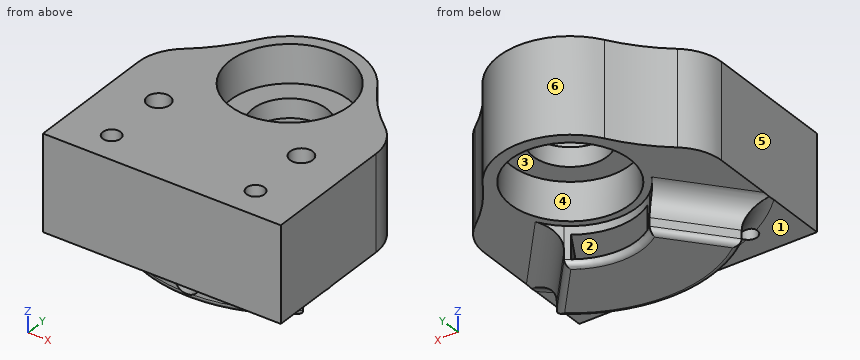
from build123d import *

# Parameters (mm, degrees)
EXTRUDE_1_DEPTH          = 4
EXTRUDE_1_DEPTH_BACK     = 4
SKETCH_2_R               = 0.95
SKETCH_2_R_2             = 0.75
SKETCH_3_R               = 5
CUT_EXTRUDE_1_DEPTH      = 3.2
SKETCH_6_R               = 3.1
CUT_EXTRUDE_2_DEPTH      = 24.749526311
EXTRUDE_3_DEPTH          = 3.2
CUT_EXTRUDE_3_DEPTH      = 1.2
CUT_EXTRUDE_3_DEPTH_BACK = 0.8
SKETCH_10_R              = 0.95
EXTRUDE_4_DEPTH          = 2
FILLET_4_R               = 2
FILLET_START             = -7
FILLET_5_2_DEPTH         = 9
FILLET_START_2           = -2
FILLET_5_3_DEPTH         = 9
SKETCH_11_R              = 1.1
CUT_EXTRUDE_4_DEPTH      = 5


with BuildPart() as part:
    # 草图2 → 凸台-拉伸1 (new, two sides: drawn at the far end of the back side and taken through both)
    with BuildSketch(Plane.XY.offset(-EXTRUDE_1_DEPTH_BACK)):
        with BuildLine():
            Line((-10, 11.178983643), (-10, 0))
            Line((-10, 0), (10, 0))
            Line((10, 0), (10, 11.178983643))
            ThreePointArc((10, 11.178983643), (9.606342006, 12.909387452), (8.502851331, 14.299197613))
            ThreePointArc((8.502851331, 14.299197613), (6.641519688, 16.075059286), (5.11101252, 18.142857143))
            ThreePointArc((5.11101252, 18.142857143), (0, 21), (-5.11101252, 18.142857143))
            ThreePointArc((-5.11101252, 18.142857143), (-6.641519688, 16.075059286), (-8.502851331, 14.299197613))
            ThreePointArc((-8.502851331, 14.299197613), (-9.606342006, 12.909387452), (-10, 11.178983643))
        make_face()
        with Locations((-6, 8)):
            Circle(SKETCH_2_R, mode=Mode.SUBTRACT)
        with Locations((-6.05, 2.55)):
            Circle(SKETCH_2_R_2, mode=Mode.SUBTRACT)
        with Locations(Location((6.05, 2.55, 0), (0, 0, 180))):
            Circle(SKETCH_2_R_2, mode=Mode.SUBTRACT)
        with Locations(Location((6, 8, 0), (0, 0, 180))):
            Circle(SKETCH_2_R, mode=Mode.SUBTRACT)
    extrude(amount=EXTRUDE_1_DEPTH + EXTRUDE_1_DEPTH_BACK)

    # 草图3 → 切除-拉伸1 (cut)
    with BuildSketch(Plane.XY.offset(4)):
        with Locations((0, 15)):
            Circle(SKETCH_3_R)
    cut_extrude_1 = extrude(amount=-CUT_EXTRUDE_1_DEPTH, mode=Mode.SUBTRACT)

    # 镜向1: 切除-拉伸1 across plane
    add(cut_extrude_1.mirror(Plane.XY), mode=Mode.SUBTRACT)

    # 草图6 → 切除-拉伸2 (cut, through all)
    with BuildSketch(Plane.XY.offset(0.8)):
        with Locations((0, 15)):
            Circle(SKETCH_6_R)
    extrude(amount=-CUT_EXTRUDE_2_DEPTH, mode=Mode.SUBTRACT)

    # 草图8 → 凸台-拉伸3 (add)
    with BuildSketch(Plane(origin=(0, 0, -4), x_dir=(-1, 0, 0), z_dir=(0, 0, -1))):
        with BuildLine():
            Line((-3.599610614, 10.710151119), (-7.777730077, 5.730862238))
            ThreePointArc((-7.777730077, 5.730862238), (0, 2.9), (7.777730077, 5.730862238))
            Line((7.777730077, 5.730862238), (3.599610614, 10.710151119))
            ThreePointArc((3.599610614, 10.710151119), (0, 9.4), (-3.599610614, 10.710151119))
        make_face()
    extrude(amount=EXTRUDE_3_DEPTH)

    # 草图9 → 切除-拉伸3 (cut, two sides: drawn at the far end of the back side and taken through both)
    with BuildSketch(Plane(origin=(0, 0, -5.5), x_dir=(-1, 0, 0), z_dir=(0, 0, -1)).offset(-CUT_EXTRUDE_3_DEPTH_BACK)):
        with BuildLine():
            Line((-3.221829655, 10.419627344), (-5.977379212, 5.646875508))
            ThreePointArc((-5.977379212, 5.646875508), (0, 3.9), (5.977379212, 5.646875508))
            Line((5.977379212, 5.646875508), (3.221829655, 10.419627344))
            ThreePointArc((3.221829655, 10.419627344), (0, 9.4), (-3.221829655, 10.419627344))
        make_face()
    extrude(amount=CUT_EXTRUDE_3_DEPTH + CUT_EXTRUDE_3_DEPTH_BACK, mode=Mode.SUBTRACT)

    # 草图10 → 凸台-拉伸4 (add)
    with BuildSketch(Plane(origin=(0, 0, -4), x_dir=(-1, 0, 0), z_dir=(0, 0, -1))):
        with Locations((-6, 8)):
            Circle(SKETCH_10_R)
        with Locations(Location((6, 8, 0), (0, 0, 180))):
            Circle(SKETCH_10_R)
    extrude(amount=-EXTRUDE_4_DEPTH)

    # 圆角4
    # the kernel refuses this fillet: 2 mm, written as the material it adds along each edge
    with BuildSketch(Plane(origin=(10.991668126, 1.900640023, -4), x_dir=(0.7660444431189769, 0.6427876096865407, 0), z_dir=(-0.6427876096865407, 0.7660444431189769, 0))) as fillet_4_piece_1_section:
        with BuildLine():
            CenterArc((FILLET_4_R, FILLET_4_R), FILLET_4_R, 180, 90)
            Line((0, FILLET_4_R), (0, 0))
            Line((0, 0), (FILLET_4_R, 0))
        make_face()
    fillet_4_piece_1 = extrude(amount=16.5, mode=Mode.PRIVATE)
    fillet_4_piece_1 = fillet_4_piece_1 - Plane(origin=(0, 15, -4), x_dir=(-0.6427876096865404, -0.7660444431189772, 0), z_dir=(0, 0, 1)) * Cylinder(5.6, 42, mode=Mode.PRIVATE)
    fillet_4_piece_1 = fillet_4_piece_1 & Plane(origin=(0, 15, -4), x_dir=(0.6427876096865403, -0.7660444431189773, 0), z_dir=(0, 0, 1)) * Cylinder(12.1, 42, mode=Mode.PRIVATE)
    add(fillet_4_piece_1)
    with BuildSketch(Plane(origin=(-0.385672566, 14.540373334, -4), x_dir=(-0.766044443118977, 0.6427876096865406, 0), z_dir=(-0.6427876096865406, -0.7660444431189771, 0))) as fillet_4_piece_2_section:
        with BuildLine():
            CenterArc((FILLET_4_R, FILLET_4_R), FILLET_4_R, 180, 90)
            Line((0, FILLET_4_R), (0, 0))
            Line((0, 0), (FILLET_4_R, 0))
        make_face()
    fillet_4_piece_2 = extrude(amount=16.5, mode=Mode.PRIVATE)
    fillet_4_piece_2 = fillet_4_piece_2 - Plane(origin=(0, 15, -4), x_dir=(-0.6427876096865404, -0.7660444431189772, 0), z_dir=(0, 0, 1)) * Cylinder(5.6, 42, mode=Mode.PRIVATE)
    fillet_4_piece_2 = fillet_4_piece_2 & Plane(origin=(0, 15, -4), x_dir=(0.6427876096865403, -0.7660444431189773, 0), z_dir=(0, 0, 1)) * Cylinder(12.1, 42, mode=Mode.PRIVATE)
    add(fillet_4_piece_2)
    with BuildSketch(Plane(origin=(0, 15, -4), x_dir=(0.6427876096865403, -0.7660444431189772, 0), z_dir=(0.7660444431189772, 0.6427876096865403, 0))) as fillet_4_piece_3_section:
        with BuildLine():
            CenterArc((12.1 + FILLET_4_R, FILLET_4_R), FILLET_4_R, 180, 90)
            Line((12.1, FILLET_4_R), (12.1, 0))
            Line((12.1, 0), (12.1 + FILLET_4_R, 0))
        make_face()
    fillet_4_piece_3 = revolve(axis=Axis((0, 15, -4), (0, 0, -1)), revolution_arc=80, mode=Mode.PRIVATE)
    fillet_4_piece_3 = fillet_4_piece_3 - Plane(origin=(-6.05, 2.55, -4), x_dir=(1, 0, 0), z_dir=(0, 0, -1)) * Cylinder(0.75, 57, mode=Mode.PRIVATE)
    fillet_4_piece_3 = fillet_4_piece_3 - Plane(origin=(6.05, 2.55, -4), x_dir=(-1, 0, 0), z_dir=(0, 0, -1)) * Cylinder(0.75, 57, mode=Mode.PRIVATE)
    add(fillet_4_piece_3)
    with BuildSketch(Plane(origin=(10.991668126, 1.900640023, -4), x_dir=(0.7660444431189769, 0.6427876096865407, 0), z_dir=(-0.6427876096865407, 0.7660444431189769, 0))) as fillet_4_piece_4a_section:
        with BuildLine():
            CenterArc((FILLET_4_R, FILLET_4_R), FILLET_4_R, 180, 90)
            Line((0, FILLET_4_R), (0, 0))
            Line((0, 0), (FILLET_4_R, 0))
        make_face()
    fillet_4_piece_4a = extrude(amount=16.5, mode=Mode.PRIVATE)
    fillet_4_piece_4a = split(fillet_4_piece_4a, bisect_by=Plane(origin=(10, 1.900640023, -4), z_dir=(-1, 0, 0)), keep=Keep.TOP, mode=Mode.PRIVATE)
    fillet_4_piece_4a = fillet_4_piece_4a - Plane(origin=(0, 15, -4), x_dir=(0.6427876096865403, -0.7660444431189773, 0), z_dir=(0, 0, 1)) * Cylinder(12.1, 42, mode=Mode.PRIVATE)
    with BuildSketch(Plane(origin=(0, 15, -4), x_dir=(0.8963584591585163, -0.44333002683663375, 0), z_dir=(0.44333002683663375, 0.8963584591585163, 0))) as fillet_4_piece_4b_section:
        with BuildLine():
            CenterArc((12.1 + FILLET_4_R, FILLET_4_R), FILLET_4_R, 180, 90)
            Line((12.1, FILLET_4_R), (12.1, 0))
            Line((12.1, 0), (12.1 + FILLET_4_R, 0))
        make_face()
    fillet_4_piece_4b = revolve(axis=Axis((0, 15, -4), (0, 0, -1)), revolution_arc=103.683456225, mode=Mode.PRIVATE)
    fillet_4_piece_4b = split(fillet_4_piece_4b, bisect_by=Plane(origin=(10, 15, -4), z_dir=(-1, 0, 0)), keep=Keep.TOP, mode=Mode.PRIVATE)
    fillet_4_piece_4b = split(fillet_4_piece_4b, bisect_by=Plane(origin=(0, 15, -4), z_dir=(0.7660444431189771, 0.6427876096865406, 0)), keep=Keep.TOP, mode=Mode.PRIVATE)
    fillet_4_piece_4 = fillet_4_piece_4a & fillet_4_piece_4b
    add(fillet_4_piece_4)
    with BuildSketch(Plane(origin=(-0.385672566, 14.540373334, -4), x_dir=(-0.766044443118977, 0.6427876096865406, 0), z_dir=(-0.6427876096865406, -0.7660444431189771, 0))) as fillet_4_piece_5a_section:
        with BuildLine():
            CenterArc((FILLET_4_R, FILLET_4_R), FILLET_4_R, 180, 90)
            Line((0, FILLET_4_R), (0, 0))
            Line((0, 0), (FILLET_4_R, 0))
        make_face()
    fillet_4_piece_5a = extrude(amount=16.5, mode=Mode.PRIVATE)
    fillet_4_piece_5a = split(fillet_4_piece_5a, bisect_by=Plane(origin=(-10, 14.540373334, -4), z_dir=(1, 0, 0)), keep=Keep.TOP, mode=Mode.PRIVATE)
    fillet_4_piece_5a = fillet_4_piece_5a - Plane(origin=(0, 15, -4), x_dir=(0.6427876096865403, -0.7660444431189773, 0), z_dir=(0, 0, 1)) * Cylinder(12.1, 42, mode=Mode.PRIVATE)
    with BuildSketch(Plane(origin=(0, 15, -4), x_dir=(0.6427876096865403, -0.7660444431189772, 0), z_dir=(0.7660444431189772, 0.6427876096865403, 0))) as fillet_4_piece_5b_section:
        with BuildLine():
            CenterArc((12.1 + FILLET_4_R, FILLET_4_R), FILLET_4_R, 180, 90)
            Line((12.1, FILLET_4_R), (12.1, 0))
            Line((12.1, 0), (12.1 + FILLET_4_R, 0))
        make_face()
    fillet_4_piece_5b = revolve(axis=Axis((0, 15, -4), (0, 0, -1)), revolution_arc=103.683456225, mode=Mode.PRIVATE)
    fillet_4_piece_5b = split(fillet_4_piece_5b, bisect_by=Plane(origin=(-10, 15, -4), z_dir=(1, 0, 0)), keep=Keep.TOP, mode=Mode.PRIVATE)
    fillet_4_piece_5b = split(fillet_4_piece_5b, bisect_by=Plane(origin=(0, 15, -4), z_dir=(-0.7660444431189771, 0.6427876096865406, 0)), keep=Keep.TOP, mode=Mode.PRIVATE)
    fillet_4_piece_5 = fillet_4_piece_5a & fillet_4_piece_5b
    add(fillet_4_piece_5)

    # 圆角5: read off the stored shape, not the designer's step
    # 圆角5 outline → 圆角5 (revolve, cut)
    with BuildSketch(Plane.XZ.offset(-15)):
        with BuildLine():
            Line((12.1, -7.2), (12.1, -6.7))
            ThreePointArc((12.1, -6.7), (11.953553391, -7.053553391), (11.6, -7.2))
            Line((11.6, -7.2), (12.1, -7.2))
        make_face()
        with BuildLine():
            Line((5.6, -7.2), (6.1, -7.2))
            ThreePointArc((6.1, -7.2), (5.746446609, -7.053553391), (5.6, -6.7))
            Line((5.6, -6.7), (5.6, -7.2))
        make_face()
    revolve(axis=Axis((0, 15, 0), (0, 0, 1)), mode=Mode.SUBTRACT)

    # Fillet 5 2 outline → Fillet 5 2 (cut)
    with BuildSketch(Plane(origin=(0, 0, 0), x_dir=(0.7660444431189767, 0.6427876096865409, 0), z_dir=(0.6427876096865409, -0.7660444431189768, 0)).offset(FILLET_START)):
        with BuildLine():
            Line((9.641814145, -7.2), (9.641814145, -6.7))
            ThreePointArc((9.641814145, -6.7), (9.495367536, -7.053553391), (9.141814145, -7.2))
            Line((9.141814145, -7.2), (9.641814145, -7.2))
        make_face()
    extrude(amount=FILLET_5_2_DEPTH, mode=Mode.SUBTRACT)

    # Fillet 5 3 outline → Fillet 5 3 (cut)
    with BuildSketch(Plane(origin=(0, 0, 0), x_dir=(0.7660444431189767, -0.6427876096865409, 0), z_dir=(0.6427876096865409, 0.7660444431189768, 0)).offset(FILLET_START_2)):
        with BuildLine():
            Line((-9.641814145, 7.2), (-9.641814145, 6.7))
            ThreePointArc((-9.641814145, 6.7), (-9.495367536, 7.053553391), (-9.141814145, 7.2))
            Line((-9.141814145, 7.2), (-9.641814145, 7.2))
        make_face()
    extrude(amount=FILLET_5_3_DEPTH, mode=Mode.SUBTRACT)

    # 草图11 → 切除-拉伸4 (cut)
    with BuildSketch(Plane(origin=(0, 0, 0), x_dir=(1, 0, 0), z_dir=(0, 1, 0))):
        with Locations(Location((0, 5.7, 0), (0, 0, 65.380022671))):
            Circle(SKETCH_11_R)
    extrude(amount=CUT_EXTRUDE_4_DEPTH, mode=Mode.SUBTRACT)


solid = part.part
Can you work these out from the model? Positions are in its coordinate system, mm. Face numbers are marked on the shaded views. A direction names the side the tool comes from. Coordinates: 2 decimals unless noted, no trailing zeros. Write each loop counter-clockwise with the first axis right and the second up, starting at its lowest first coordinate (ties: lowest second). Pieces come first, ordered by that corner, then holes.
Q1. Please list where these lines run through material, in increasing order: L1, parallel to X at y = 8, z = 0; L2, parallel to Y at x = 0, z = -1.9; L3, parallel to Z at x = 2.5, y = 8.
Results found:
L1: x = -10 to -6.95, -5.05 to 5.05, 6.95 to 10
L2: y = 0 to 10, 20 to 21
L3: z = -7.2 to -6.7, -4.7 to 4
Q2. Imagine slicing it at C-C, the plane z = 0.25. List the corners of the cut face in (x, y) for me.
Results found:
outline: (-10, 0) - (10, 0) - (10, 11.18) arc R4 ccw to (8.5, 14.3) arc R15 cw to (5.11, 18.14) arc R6 ccw to (-5.11, 18.14) arc R15 cw to (-8.5, 14.3) arc R4 ccw to (-10, 11.18) - close; hole circle Ø1.9 at (-6, 8); hole circle Ø1.5 at (-6.05, 2.55); hole circle Ø6.2 at (0, 15); hole circle Ø1.9 at (6, 8); hole circle Ø1.5 at (6.05, 2.55)
Q3. Imagine slicing it at B-B, the plane z = -2.25. List the corners of the cut face in (x, y) for me, plus the area to 3 significant figures.
Results found:
outline: (-10, 0) - (10, 0) - (10, 11.18) arc R4 ccw to (8.5, 14.3) arc R15 cw to (5.11, 18.14) arc R6 ccw to (-5.11, 18.14) arc R15 cw to (-8.5, 14.3) arc R4 ccw to (-10, 11.18) - close; hole circle Ø1.5 at (-6.05, 2.55); hole circle Ø10 at (0, 15); hole circle Ø1.5 at (6.05, 2.55)
area: 273 mm2
Q4. Imagine slicing it at D-D, the plane x = 0. List the corners of the cut face in (y, z) for me.
Results found:
outline: (0, -4) - (0.9, -4) arc R2 cw to (2.33, -4.6) - (5, -4.6) - (5, -4.7) - (9.4, -4.7) - (9.4, -4) - (10, -4) - (10, -0.8) - (11.9, -0.8) - (11.9, 0.8) - (10, 0.8) - (10, 4) - (0, 4) - close; (2.91, -6.8) arc R0.5 ccw to (3.4, -7.2) - (8.9, -7.2) arc R0.5 ccw to (9.4, -6.7) - (5, -6.7) - (5, -6.8) - close; (18.1, -0.8) - (20, -0.8) - (20, -4) - (21, -4) - (21, 4) - (20, 4) - (20, 0.8) - (18.1, 0.8) - close
Q5. Which directions (+Z, -Z, +X, -X, +Y, -Y) give clear straight access to the entire face, cutting with the end or side of a thin tool? Please do the marked faces 1, 2 and 3.
Results found:
face 1: -Z, -Y
face 2: none
face 3: -Z
Q6. For P1, Ø1.5, axis at x = -4.5, z = -4, coming from the +Y side; P2, Ø3, axis at x = 0, y = 12.5, coming from the -Z side; P3, Ø1.5, axis at x = -3, y = 2, coming from the -Z side, each with a flat end and sliding along its axis, tell me the tip position at first contact or that it passes through.
Results found:
P1: stops at y = 19.68
P2: stops at z = -0.8
P3: stops at z = -4.69
Q7. Imagine slicing it at A-A, the plane y = 15. List the corners of the cut face in (x, z) for me.
Results found:
outline: (-7.69, -4) - (-5, -4) - (-5, -0.8) - (-3.1, -0.8) - (-3.1, 0.8) - (-5, 0.8) - (-5, 4) - (-7.69, 4) - close; (3.1, -0.8) - (5, -0.8) - (5, -4) - (7.69, -4) - (7.69, 4) - (5, 4) - (5, 0.8) - (3.1, 0.8) - close
Q8. If we mould it in two halves opening along Y, with no side actions, what happens to the marked faces 4, 5 and 6? For each: +Y half, -Y half, draft (parallel to the pull), parting line (faces both ways), or undercut.
Results found:
face 4: undercut
face 5: draft
face 6: +Y half
